Could you check a few things on this model? Use its own coordinates, in mm. A direction names the side the tool comes from. Give positions to 0.01 mm unless a question says otherwise; leave off trailing zeros. Loops run counter-clockwise (first coordinate to the right, second up) from the corner with the lowest first, then second, coordinate; pieces in that order, holes last. Notation, with made-up numbers: (89.25, 84) - (133.25, 84) arc R19 cw to (133.25, 99) - close; hole circle Ø11 at (12.5, -17.5). An arc over 180 degrees is marked (long way). Answer in a Markdown table with one row per item. Add a question column.
```python
from build123d import *

# Parameters (mm, degrees)
F0_W     = 400
F0_H     = 404.9209267448
F1_DEPTH = 40
F2_R     = 43.4558441227
F3_W     = 40
F3_H     = 40
F4_DEPTH = 360
F5_R     = 7.24
F6_W     = 40
F6_H     = 40
F7_DEPTH = 360
F8_R     = 7.2426406871
F9_R     = 5


with BuildPart() as f1:
    # F0 (on Top) → F1 (new body)
    with BuildSketch(Plane.XY):
        with Locations((65.5444227159, 0)):
            Rectangle(F0_W, F0_H)
    extrude(amount=F1_DEPTH)

    # F2
    f2_edges = [f1.edges().sort_by_distance(p)[0] for p in [
        (-134.455577, -202.460463, 20),
        (-134.455577, 202.460463, 20),
        (265.544423, 202.460463, 20),
        (265.544423, -202.460463, 20),
    ]]
    fillet(f2_edges, radius=F2_R)

    # F3 (on Top) → F4 (join)
    with BuildSketch(Plane.XY):
        with Locations((-74.4555772841, -142.4604633724)):
            Rectangle(F3_W, F3_H)
    extrude(amount=F4_DEPTH)

    # F5
    f5_edges = [f1.edges().sort_by_distance(p)[0] for p in [
        (-54.455577, -162.460463, 200),
        (-54.455577, -122.460463, 200),
        (-94.455577, -122.460463, 200),
        (-94.455577, -162.460463, 200),
    ]]
    fillet(f5_edges, radius=F5_R)

    # F6 (on Top) → F7 (join)
    with BuildSketch(Plane.XY):
        with Locations((205.5444227159, -142.4604633724)):
            Rectangle(F6_W, F6_H)
        with Locations((205.5444227159, 142.4604633724)):
            Rectangle(F6_W, F6_H)
        with Locations((-74.4555772841, 142.4604633724)):
            Rectangle(F6_W, F6_H)
    extrude(amount=F7_DEPTH)

    # F8
    f8_edges = [f1.edges().sort_by_distance(p)[0] for p in [
        (-54.455577, 162.460463, 200),
        (-94.455577, 162.460463, 200),
        (-94.455577, 122.460463, 200),
        (-54.455577, 122.460463, 200),
        (225.544423, 122.460463, 200),
        (225.544423, 162.460463, 200),
        (185.544423, 122.460463, 200),
        (185.544423, 162.460463, 200),
        (225.544423, -162.460463, 200),
        (225.544423, -122.460463, 200),
        (185.544423, -162.460463, 200),
        (185.544423, -122.460463, 200),
    ]]
    fillet(f8_edges, radius=F8_R)

    # F9
    f9_edges = [f1.edges().sort_by_distance(p)[0] for p in [
        (265.544423, 0, 0),
        (252.816501, 189.732541, 0),
        (65.544423, 202.460463, 0),
        (-121.727655, 189.732541, 0),
        (-134.455577, 0, 0),
        (-121.727655, -189.732541, 0),
        (65.544423, -202.460463, 0),
        (252.816501, -189.732541, 0),
    ]]
    fillet(f9_edges, radius=F9_R)


solid = f1.part
```
(1) For pin 1 Ø6 at (x, z) = (-89.5, 227) entering from +Y; pin 2 Ø20.5 at (y, z) = (146, 213) entering from -X; pin 3 Ø20.5 at (y, z) = (-141.5, 189.5) entering from +X, each with a flat end and sliding along its axis, tell me the tip position at first contact or that it passes through.
(2) I want a section at C-C on x = 100. Please give me the cut outline in (y, z).
(3) I want a section at D-D on y = -1.5. Please give me the cut outline in (x, z), then the cut area to 3 significant figures.
(4) On a 3-axis mill with a long thin cutter (end or side, diameter ignored), from which of +Z, -Z, +X, -X, +Y, -Y can I reach the whole of each face in a straight line? I mean faces 4 (the flat face through (205, 143, 360)), 5 (the flat face through (63, 3, 0)), 6 (the flat face through (205, -122.46, 198)), 7 (the flat face through (-94.456, 142, 198)), 8 (the flat face through (-54.456, 142, 198)). Say none if no direction works.
(5) I want a section at B-B on y = -141. Please give me the cut outline in (x, z), then the cut area to 3 significant figures.
(6) I want a section at A-A on z = 207. State how many separate pieces and enclosed holes the cut face has, then the cut area to 3 significant figures.
(7) Please list where these lines run through material, in increasing order: line 1 (Y direction, x = -84, z = 294.5); line 2 (X direction, y = 132.5, z = 184); line 3 (Z direction, x = 152.5, y = 48).
(8) We'd pull the mould along Y, two halves only. Please class faces 1 (the flat face through (205, 122.46, 198)), 2 (the flat face through (-75, -162.46, 198)), 3 (the flat face through (-54.456, -143, 198)): pulls with the +Y half, pulls with the -Y half, needs draft (parallel to the pull), parting line crosses it, or undercut.
Reported:
| question | item | result |
|---|---|---|
| 1 | pin 1 | y = 162.46 |
| 1 | pin 2 | x = -94.46 |
| 1 | pin 3 | x = 225.54 |
| 2 | outline | (-202.46, 5) arc R5 ccw to (-197.46, 0) - (197.46, 0) arc R5 ccw to (202.46, 5) - (202.46, 40) - (-202.46, 40) - close |
| 3 | outline | (-134.46, 5) arc R5 ccw to (-129.46, 0) - (260.54, 0) arc R5 ccw to (265.54, 5) - (265.54, 40) - (-134.46, 40) - close |
| 3 | area | 16,000 mm² |
| 4 | face 4 | +Z, +X, -X, +Y, -Y |
| 4 | face 5 | -Z, +X, -X, +Y, -Y |
| 4 | face 6 | +Z, +X, -X |
| 4 | face 7 | +Z, -X, +Y, -Y |
| 4 | face 8 | +Z, +Y, -Y |
| 5 | outline | (-134.46, 5) arc R5 ccw to (-129.46, 0) - (260.54, 0) arc R5 ccw to (265.54, 5) - (265.54, 40) - (225.54, 40) - (225.54, 360) - (185.54, 360) - (185.54, 40) - (-54.46, 40) - (-54.46, 360) - (-94.46, 360) - (-94.46, 40) - (-134.46, 40) - close |
| 5 | area | 41,600 mm² |
| 6 | separate pieces | 4 |
| 6 | enclosed holes | 0 |
| 6 | area | 6,220 mm² |
| 7 | line 1 | -162.46 to -122.46, 122.46 to 162.46 |
| 7 | line 2 | -94.46 to -54.46, 185.54 to 225.54 |
| 7 | line 3 | 0 to 40 |
| 8 | face 1 | undercut |
| 8 | face 2 | pulls with the -Y half |
| 8 | face 3 | needs draft |
